Answer from the drawing. Dimensions are ordinates in mm from the lowest x, y and z of the part. Give positions to 0.01 mm unless a question says otherwise; leave off trailing zeros. Loops run counter-clockwise (first coordinate to the right, second up) from the corner with the lowest first, then second, coordinate; pieces in that order, holes last. Notation, with made-up numbers: M 70,18.5 L 126,18.5 A31 ccw 126,48.5 Z; hole C 37.5,-2.75 d1. An arc over 180 degrees is marked long. Use a Markdown table: item, result.
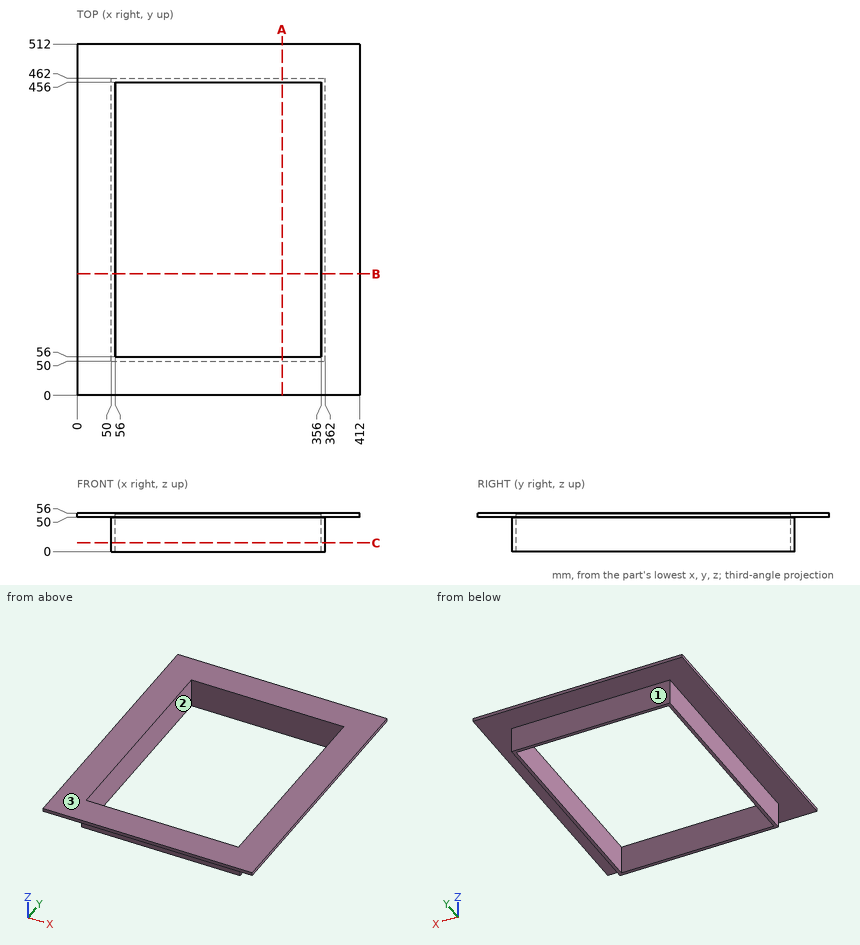
(1) A cutting plane is placed at C-C (z = 13). Write down the section's boundary in (x, y), and give its area (3 significant figures).
Entries:
| item | result |
|---|---|
| outline | M 50,50 L 362,50 L 362,462 L 50,462 Z; hole M 56,56 L 356,56 L 356,456 L 56,456 Z |
| area | 8,540 mm² |
(2) Consider probe 1 along X at (y, z) = (299, 3); probe 2 along X at (y, z) = (114.5, 53.5); probe 3 along Y at (x, z) = (298, 20.5). Determine where each line is inside the solid, lowest interval first. Write a range as [from, to].
Entries:
| item | result |
|---|---|
| probe 1 | x = [50, 56], [356, 362] |
| probe 2 | x = [0, 56], [356, 412] |
| probe 3 | y = [50, 56], [456, 462] |
(3) Given P1, Ø17, axis at x = 281, z = 31, coming from the -Y side; P2, Ø1, axis at x = 246.5, z = 5.5, coming from the +Y side; P3, Ø15, axis at y = 221, z = 12.5, coming from the -X side; P4, Ø10, axis at x = 302, y = 448.5, coming from the -Z side, each flat-ended and moving along its own axis, determine where each tip first touches the part or whether it passes through.
Entries:
| item | result |
|---|---|
| P1 | stops at y = 50 |
| P2 | stops at y = 462 |
| P3 | stops at x = 50 |
| P4 | passes through |
(4) A cutting plane is placed at B-B (y = 177). Write down the section's boundary in (x, z), and give its area (3 significant figures).
Entries:
| item | result |
|---|---|
| outline | M 0,50 L 50,50 L 50,0 L 56,0 L 56,56 L 0,56 Z; M 356,0 L 362,0 L 362,50 L 412,50 L 412,56 L 356,56 Z |
| area | 1,270 mm² |
(5) The mould has two halves that part along Y. Classify the marked faces 1, 2 and 3: released by +Y, released by -Y, zero draft, split by the parting line, or undercut.
Entries:
| item | result |
|---|---|
| face 1 | released by +Y |
| face 2 | undercut |
| face 3 | zero draft |
(6) A cutting plane is placed at A-A (x = 299). Write down the section's boundary in (y, z).
Entries:
| item | result |
|---|---|
| outline | M 0,50 L 50,50 L 50,0 L 56,0 L 56,56 L 0,56 Z; M 456,0 L 462,0 L 462,50 L 512,50 L 512,56 L 456,56 Z |
